from build123d import *

# Parameters (mm, degrees)
F0_R     = 12.7
F0_R_2   = 8.2296
F1_DEPTH = 2.286
F2_DEPTH = 12.7
F3_W     = 6.35
F3_H     = 35.38055
F4_DEPTH = 12.7


with BuildPart() as f1:
    # F0 (on Top) → F1 (new body)
    with BuildSketch(Plane.XY):
        Circle(F0_R)
        Circle(F0_R_2, mode=Mode.SUBTRACT)
        Circle(F0_R_2)
    extrude(amount=-F1_DEPTH)

    # F0 (on Top) → F2 (join)
    with BuildSketch(Plane.XY):
        Circle(F0_R)
        Circle(F0_R_2, mode=Mode.SUBTRACT)
    extrude(amount=F2_DEPTH)

    # F3 (on face) → F4 (cut, through all)
    with BuildSketch(Plane.XY.offset(12.7)):
        Rectangle(F3_W, F3_H)
    extrude(amount=-F4_DEPTH, mode=Mode.SUBTRACT)


solid = f1.part
The model under review builds one solid part; all positions refer to its coordinate system, in mm. A direction names the side the tool comes from. Give positions to 0.01 mm unless a question says otherwise; leave off trailing zeros. Write each loop counter-clockwise with the first axis right and the second up, starting at its lowest first coordinate (ties: lowest second). Pieces come first, ordered by that corner, then holes. Notation, with made-up numbers: M 3,4.25 L 25,4.25 A21 ccw 25,35.25 Z; hole C 87,88 d5. An arc over 180 degrees is marked long. One line per question, with ' | ' between items. Start each with the question number.
Item 1: We need section D-D on y = 2. Write out the cut boundary in (x, z).
Item 2: Wall thickness on line 1 (Z direction, x = -7, y = -0.5); line 2 (X direction, y = 4, z = 2.5); line 3 (X direction, y = 5, z = 1.75): over which ranges is each line inside the solid? List them lowest first. Write a range as from..to.
Item 3: For faces 4 (the flat face through (3.175, -10, 6)), 5 (the cylindrical face through (-8.23, 0.14, 6.26)), 6 (the flat face through (9, 0, 12.7)), list the 3-axis set-ups (+Z, -Z, +X, -X, +Y, -Y) from which the entire face can be reached by the end or side of a thin tool; tool diameter is ignored.
Item 4: Draft analysis for pull direction Y (two halves, no side actions). For faces 1 (the flat face through (0, 0, 0)), 2 (the cylindrical face through (12.114, 3.815, 5.102)), 3 (the flat face through (-3.175, 10, 6)), state which applies: released by +Y, released by -Y, zero draft, split by the parting line, or undercut.
Item 5: We need section B-B on y = -2.25. Write out the cut boundary in (x, z), plus the area to 3 significant figures.
Item 6: We need section C-C on x = 1.5. Write out the cut boundary in (y, z), plus the area to 3 significant figures.
Item 7: We need section A-A on z = 2.5. Write out the cut boundary in (x, y) (3 decimals), plus the area to 3 significant figures.
Item 8: For pin 1 (1 mm diameter, centred on x = -7.5, z = 10, fed in from -Y); pin 2 (8 mm diameter, centred on x = -2, y = 2, fed in from +Z); pin 3 (8 mm diameter, centred on x = -5, z = -0.5, fed in from +Y), all flat-tipped, find the tip position at first contact; note any pin that passes through.
Results found:
1) outline: M -12.54,-2.29 L 12.54,-2.29 L 12.54,12.7 L 7.98,12.7 L 7.98,0 L -7.98,0 L -7.98,12.7 L -12.54,12.7 Z
2) line 1: z = -2.29..0 | line 2: x = -12.05..-7.19, 7.19..12.05 | line 3: x = -11.67..-6.54, 6.54..11.67
3) face 4: +Z, +Y, -Y | face 5: +Z | face 6: +Z, +X, -X, +Y, -Y
4) face 1: undercut | face 2: split by the parting line | face 3: zero draft
5) outline: M -12.5,-2.29 L 12.5,-2.29 L 12.5,12.7 L 7.92,12.7 L 7.92,0 L -7.92,0 L -7.92,12.7 L -12.5,12.7 Z | area: 174 mm2
6) outline: M -12.61,-2.29 L 12.61,-2.29 L 12.61,0 L -12.61,0 Z | area: 57.7 mm2
7) outline: M -3.175,-12.297 L -3.175,-7.592 A8.23 cw -3.175,7.592 L -3.175,12.297 A12.7 ccw Z; M 3.175,-12.297 A12.7 ccw 3.175,12.297 L 3.175,7.592 A8.23 cw 3.175,-7.592 Z | area: 236 mm2
8) pin 1: stops at y = -10.6 | pin 2: stops at z = 0 | pin 3: stops at y = 12.66
